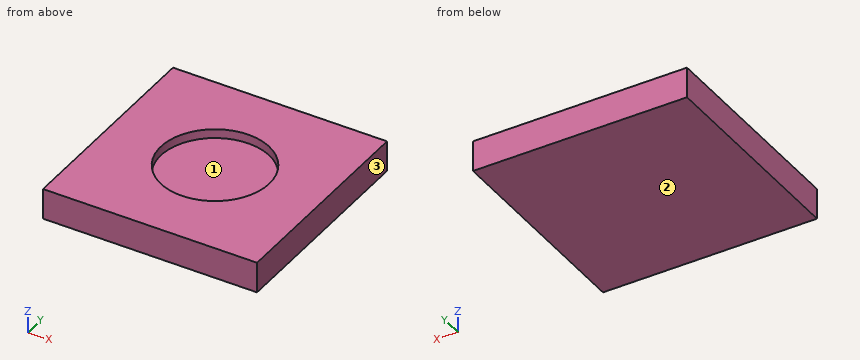
from build123d import *

# Parameters (mm, degrees)
SKETCH1_W           = 49.4
SKETCH1_H           = 49.4
SKETCH1_R           = 12.5
BOSS_EXTRUDE1_DEPTH = 7.1
SKETCH5_R           = 12.5
BOSS_EXTRUDE2_DEPTH = 5


with BuildPart() as part:
    # Sketch1 → Boss-Extrude1 (new body)
    with BuildSketch(Plane.XY):
        with Locations((24.7, 24.7)):
            Rectangle(SKETCH1_W, SKETCH1_H)
        with Locations((24.7, 24.7)):
            Circle(SKETCH1_R, mode=Mode.SUBTRACT)
    extrude(amount=BOSS_EXTRUDE1_DEPTH)

    # Sketch5 → Boss-Extrude2 (add)
    with BuildSketch(Plane(origin=(0, 0, 0), x_dir=(-1, 0, 0), z_dir=(0, 0, -1))):
        with Locations((-24.7, 24.7)):
            Circle(SKETCH5_R)
    extrude(amount=-BOSS_EXTRUDE2_DEPTH)


solid = part.part
The model under review builds one solid part; all positions refer to its coordinate system, in mm. Face numbers are marked on the shaded views. Give positions to 0.01 mm unless a question says otherwise; leave off trailing zeros. Loops run counter-clockwise (first coordinate to the right, second up) from the corner with the lowest first, then second, coordinate; pieces in that order, holes last. Notation, with made-up numbers: (86.5, -6.5) -> (128.5, -6.5) arc R16 cw to (128.5, 7.5) -> close; hole circle Ø2 at (38.25, 5.5). An arc over 180 degrees is marked (long way). Answer as a JSON object with one key per item and string values. Group by question number.
Q1. Draft analysis for pull direction X (two halves, no side actions). For the marked faces 1, 2 and 3, state which applies: pulls with the +X half, pulls with the -X half, needs draft (parallel to the pull), parting line crosses it, or undercut.
Q2. Insertion check: pin 1 (7.5 mm diameter, centred on x = 26, y = 28.5, fed in from +Z). The pin has a flat end and moves straight along its axis. Give the tip position at first contact, or say it passes through.
Q3. Take a section at B-B (y = 24.7). Write out the cut boundary in (x, z), plus the area to 3 significant figures.
Q4. Take a section at A-A (x = 13). Write out the cut boundary in (y, z), plus the area to 3 significant figures.
Q5. Wall thickness on line 1 along Y through (x, z) = (24.7, 6.3); line 2 along Z through (x, y) = (26.5, 36): over which ranges is each line inside the solid? List them lowest first.
Answer below:
{
 "1": {"face 1": "undercut", "face 2": "needs draft", "face 3": "pulls with the +X half"},
 "2": {"pin 1": "stops at z = 5"},
 "3": {"outline": "(0, 0) -> (49.4, 0) -> (49.4, 7.1) -> (37.2, 7.1) -> (37.2, 5) -> (12.2, 5) -> (12.2, 7.1) -> (0, 7.1) -> close", "area": "298 mm2"},
 "4": {"outline": "(0, 0) -> (49.4, 0) -> (49.4, 7.1) -> (29.1, 7.1) -> (29.1, 5) -> (20.3, 5) -> (20.3, 7.1) -> (0, 7.1) -> close", "area": "332 mm2"},
 "5": {"line 1": "y = 0 to 12.2, 37.2 to 49.4", "line 2": "z = 0 to 5"}
}
